```python
from build123d import *

# Parameters (mm, degrees)
SKETCH_1_R      = 2.5
EXTRUDE_1_DEPTH = 3
FILLET_1_R      = 0.5


with BuildPart() as part:
    # ｽｹｯﾁ1 → ﾎﾞｽ - 押し出し1 (new body)
    with BuildSketch(Plane.XY):
        Polygon((-12.15, 6.6), (-15, 6.6), (-15, -3.8), (-9, -3.8), (-9, -5.8), (-15, -5.8), (-15, -12), (-6, -12), (-6, -10), (-4, -10), (-4, -12), (4, -12), (4, -10), (6, -10), (6, -12), (15, -12), (15, 6.6), (12.15, 6.6), (12.15, 4.6), (10.15, 4.6), (10.15, 6.6), (-10.15, 6.6), (-10.15, 4.6), (-12.15, 4.6), align=None)
        Circle(SKETCH_1_R, mode=Mode.SUBTRACT)
    extrude(amount=EXTRUDE_1_DEPTH)

    # ﾌｨﾚｯﾄ1
    fillet_1_edges = [part.edges().sort_by_distance(p)[0] for p in [
        (-15, 6.6, 1.5),
        (15, 6.6, 1.5),
    ]]
    fillet(fillet_1_edges, radius=FILLET_1_R)


solid = part.part
```
The listing builds one solid part. Answer for the finished solid, in the listing's coordinates (mm). A direction names the side the tool comes from. Coordinates: 2 decimals unless noted, no trailing zeros. Order: outer loops, then holes, each group sorted by start corner. A loop starts at its lowest first (then second) coordinate and runs counter-clockwise, first axis right, second up. Notation, with made-up numbers: M -13.75,-17.5 L 16.25,-17.5 A22 cw 16.25,-5.5 Z; hole C 18,8.5 d9. An arc over 180 degrees is marked long. Answer as a JSON object with one key per item and string values. Group by question number.
1. Section B-B on y = 0 is taken. Write down the section's boundary in (x, z), then the cut area to 3 significant figures.
2. Straight lines are drawn through the part: line 1 (X direction, y = 5.25, z = 1.95); line 2 (X direction, y = -10.25, z = 0.35); line 3 (Y direction, x = 0, z = 1.1). For each, find the intervals that lie inside material, in ascending order.
3. Section A-A on x = 0 is taken. Write down the section's boundary in (y, z).
4. Section D-D on y = -5.5 is taken. Write down the section's boundary in (x, z).
5. A tool of negligible diameter and unlimited length cuts with its end or side. For faces 1 (the flat face through (12.15, 6, 1)), 2 (the flat face through (0, -12, 1)), 3 (the flat face through (-5, -10, 1)), from which of +Z, -Z, +X, -X, +Y, -Y can it reach the whole face along a straight path? Write none if from no direction.
6. Section C-C on z = 2.55 is taken. Write down the section's boundary in (x, y), then the cut area to 3 significant figures.
7. Determine the mould class of faces 4 (the flat face through (10, -12, 1)), 5 (the flat face through (-12, -3.8, 1)), 6 (the flat face through (-13, 6.6, 1)), 7 (the cylindrical face through (-0.54, -2.44, 1.48)) for opening direction Y: released by +Y, released by -Y, zero draft, split by the parting line, or undercut.
8. Flat-ended cylindrical pins translate along their axes: P1, Ø0.6, axis at x = -4.5, z = 1, coming from the -Y side; P2, Ø1, axis at y = -5, z = 1.5, coming from the -X side; P3, Ø3, axis at x = 0, y = 0, coming from the -Z side; P4, Ø0.6, axis at x = -11, z = 1, coming from the +Y side. Find the tip coordinate at first contact, or state that the pin passes through.
Values follow:
{
 "1": {"outline": "M -15,0 L -2.5,0 L -2.5,3 L -15,3 Z; M 2.5,0 L 15,0 L 15,3 L 2.5,3 Z", "area": "75.0 mm2"},
 "2": {"line 1": "-15 to -12.15, -10.15 to 10.15, 12.15 to 15", "line 2": "-15 to -6, -4 to 4, 6 to 15", "line 3": "-12 to -2.5, 2.5 to 6.6"},
 "3": {"outline": "M -12,0 L -2.5,0 L -2.5,3 L -12,3 Z; M 2.5,0 L 6.6,0 L 6.6,3 L 2.5,3 Z"},
 "4": {"outline": "M -9,0 L 15,0 L 15,3 L -9,3 Z"},
 "5": {"face 1": "+Z, -Z, +Y", "face 2": "+Z, -Z, +X, -X, -Y", "face 3": "+Z, -Z, -Y"},
 "6": {"outline": "M -15,-12 L -6,-12 L -6,-10 L -4,-10 L -4,-12 L 4,-12 L 4,-10 L 6,-10 L 6,-12 L 15,-12 L 15,6.1 A0.5 ccw 14.5,6.6 L 12.15,6.6 L 12.15,4.6 L 10.15,4.6 L 10.15,6.6 L -10.15,6.6 L -10.15,4.6 L -12.15,4.6 L -12.15,6.6 L -14.5,6.6 A0.5 ccw -15,6.1 L -15,-3.8 L -9,-3.8 L -9,-5.8 L -15,-5.8 Z; hole C 0,0 d5", "area": "510 mm2"},
 "7": {"face 4": "released by -Y", "face 5": "undercut", "face 6": "released by +Y", "face 7": "undercut"},
 "8": {"P1": "y = -10", "P2": "x = -9", "P3": "through", "P4": "y = 4.6"}
}
